Here's how the part is built. I have some questions about the finished solid (model axes, mm). Face numbers are marked on the shaded views. A direction names the side the tool comes from. Coordinates: 2 decimals unless noted, no trailing zeros. Write each loop counter-clockwise with the first axis right and the second up, starting at its lowest first coordinate (ties: lowest second). Pieces come first, ordered by that corner, then holes.
Item 1: I want a section at A-A (z = -19). Count the separate pieces of the cut face and the enclosed holes in it, and give its area (3 significant figures).
Item 2: I want a section at B-B (x = 41.15). Please give me the cut outline in (y, z), and give its area (3 significant figures).
Item 3: Please list where these lines run through material, in increasing order: line 1 (X direction, y = -2, z = -15.5); line 2 (X direction, y = 14, z = 1.5); line 3 (Z direction, x = 112, y = 10).
Item 4: I'm going to push flat-ended pins straight in: P1, Ø2, axis at y = 11.5, z = 4, coming from the +X side; P2, Ø2, axis at y = 13, z = -3.5, coming from the -X side; P3, Ø7, axis at y = -7.79, z = 4.5, coming from the -X side; P4, Ø2.5, axis at x = 25.65, y = -15.5, coming from the +Z side. Where does each tip first touch, or does it pass through?
Item 5: If we mould it in two halves opening along Y, with no side actions, what happens to the marked faces 1, 2, 3 and 4? For each: pulls with the +Y half, pulls with the -Y half, needs draft (parallel to the pull), parting line crosses it, or undercut.
Item 6: For the marked faces 5, 6 and 7, which set-ups out of +Z, -Z, +X, -X, +Y, -Y let a thin tool reach every point of the face, with its end or its side?
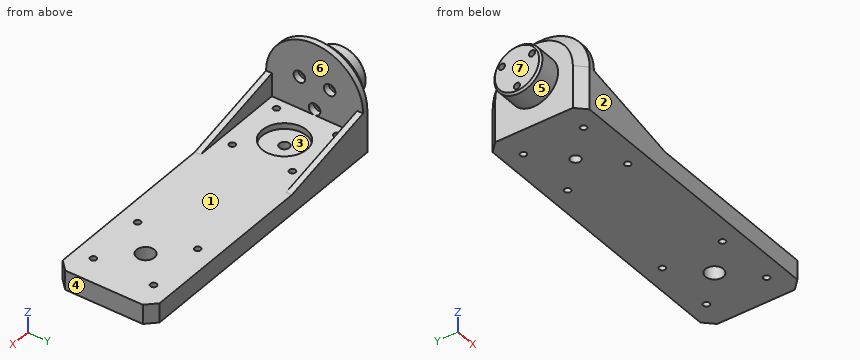
from build123d import *

# Parameters (mm, degrees)
SKETCH_2_R          = 12.4
SKETCH_2_R_2        = 1.6
EXTRUDE_1_DEPTH     = 20
EXTRUDE_2_DEPTH     = 8
SKETCH_5_W          = 155.81
SKETCH_5_H          = 50
EXTRUDE_3_DEPTH     = 10
SKETCH_6_R          = 1.6
SKETCH_6_R_2        = 2.6
SKETCH_6_R_3        = 4.6
CUT_EXTRUDE_1_DEPTH = 10
SKETCH_7_R          = 3
CUT_EXTRUDE_2_DEPTH = 3.3
SKETCH_8_R          = 11.5
CUT_EXTRUDE_3_DEPTH = 3
EXTRUDE_4_DEPTH     = 3
EXTRUDE_5_DEPTH     = 3
CHAMFER_1_SIZE      = 5
CHAMFER_2_SIZE      = 1


with BuildPart() as part:
    # 草图2 → 凸台-拉伸1 (new body)
    with BuildSketch(Plane(origin=(0, 0, 0), x_dir=(0, 0, -1), z_dir=(1, 0, 0))):
        Circle(SKETCH_2_R)
        with Locations((9, 0)):
            Circle(SKETCH_2_R_2, mode=Mode.SUBTRACT)
        with Locations((-4.5, -7.794228634)):
            Circle(SKETCH_2_R_2, mode=Mode.SUBTRACT)
        with Locations((-4.5, 7.794228634)):
            Circle(SKETCH_2_R_2, mode=Mode.SUBTRACT)
    extrude(amount=EXTRUDE_1_DEPTH)

    # 草图3 → 凸台-拉伸2 (add)
    with BuildSketch(Plane(origin=(20, 0, 0), x_dir=(0, 0, -1), z_dir=(1, 0, 0))):
        with BuildLine():
            Line((12, 25), (0, 25))
            ThreePointArc((0, 25), (-25, 0), (0, -25))
            Line((0, -25), (12, -25))
            Line((12, -25), (12, -3.12409987))
            ThreePointArc((12, -3.12409987), (-12.4, 0), (12, 3.12409987))
            Line((12, 3.12409987), (12, 25))
        make_face()
    extrude(amount=-EXTRUDE_2_DEPTH)

    # 草图5 → 凸台-拉伸3 (add)
    with BuildSketch(Plane(origin=(0, 0, -12), x_dir=(-1, 0, 0), z_dir=(0, 0, -1))):
        with Locations((-89.905, 0)):
            Rectangle(SKETCH_5_W, SKETCH_5_H)
    extrude(amount=EXTRUDE_3_DEPTH)

    # 草图6 → 切除-拉伸1 (cut)
    with BuildSketch(Plane.XY.offset(-12)):
        with Locations((25.65, 15.5)):
            Circle(SKETCH_6_R)
        with Locations((56.65, 15.5)):
            Circle(SKETCH_6_R)
        with Locations((56.65, -15.5)):
            Circle(SKETCH_6_R)
        with Locations((25.65, -15.5)):
            Circle(SKETCH_6_R)
        with Locations((41.15, 0)):
            Circle(SKETCH_6_R_2)
        with Locations((138.66, 0)):
            Circle(SKETCH_6_R_3)
        with Locations((123.16, 15.5)):
            Circle(SKETCH_6_R)
        with Locations((154.16, 15.5)):
            Circle(SKETCH_6_R)
        with Locations((154.16, -15.5)):
            Circle(SKETCH_6_R)
        with Locations((123.16, -15.5)):
            Circle(SKETCH_6_R)
    extrude(amount=-CUT_EXTRUDE_1_DEPTH, mode=Mode.SUBTRACT)

    # 草图7 → 切除-拉伸2 (cut)
    with BuildSketch(Plane(origin=(20, 0, 0), x_dir=(0, 0, -1), z_dir=(1, 0, 0))):
        with Locations((-4.5, 7.794228634)):
            Circle(SKETCH_7_R)
        with Locations((9, 0)):
            Circle(SKETCH_7_R)
        with Locations((-4.5, -7.794228634)):
            Circle(SKETCH_7_R)
    extrude(amount=-CUT_EXTRUDE_2_DEPTH, mode=Mode.SUBTRACT)

    # 草图8 → 切除-拉伸3 (cut)
    with BuildSketch(Plane.XY.offset(-12)):
        with Locations((41.15, 0)):
            Circle(SKETCH_8_R)
    extrude(amount=-CUT_EXTRUDE_3_DEPTH, mode=Mode.SUBTRACT)

    # 草图10 → 凸台-拉伸4 (add)
    with BuildSketch(Plane.XZ.offset(25)):
        Polygon((20, 0), (70, -12), (20, -12), align=None)
    extrude(amount=-EXTRUDE_4_DEPTH)

    # 草图11 → 凸台-拉伸5 (add)
    with BuildSketch(Plane(origin=(0, 25, 0), x_dir=(1, 0, 0), z_dir=(0, 1, 0))):
        Polygon((20, 0), (70, 12), (20, 12), align=None)
    extrude(amount=-EXTRUDE_5_DEPTH)

    # 倒角1
    chamfer_1_edges = [part.edges().sort_by_distance(p)[0] for p in [
        (12, 0, 25),
        (12, 25, -11),
        (12, -25, -11),
        (167.81, 25, -17),
        (167.81, -25, -17),
    ]]
    chamfer(chamfer_1_edges, length=CHAMFER_1_SIZE)

    # 倒角2
    chamfer_2_edges = [part.edges().sort_by_distance(p)[0] for p in [
        (0, 0, 12.4),
    ]]
    chamfer(chamfer_2_edges, length=CHAMFER_2_SIZE)


solid = part.part
Answer:
1. separate pieces: 1
1. enclosed holes: 10
1. area: 7,590 mm2
2. outline: (-25, -22) - (-2.6, -22) - (-2.6, -15) - (-11.5, -15) - (-11.5, -12) - (-22, -12) - (-22, -5.08) - (-25, -5.08) - close; (2.6, -22) - (25, -22) - (25, -5.08) - (22, -5.08) - (22, -12) - (11.5, -12) - (11.5, -15) - (2.6, -15) - close
2. area: 436 mm2
3. line 1: x = 12 to 39.49, 42.81 to 134.52, 142.8 to 167.81
3. line 2: x = 12 to 20
3. line 3: z = -22 to -12
4. P1: stops at x = 20
4. P2: stops at x = 12
4. P3: stops at x = 0
4. P4: passes through
5. face 1: undercut
5. face 2: pulls with the -Y half
5. face 3: undercut
5. face 4: needs draft
6. face 5: -X
6. face 6: +Z, +X
6. face 7: +Z, -Z, -X, +Y, -Y
